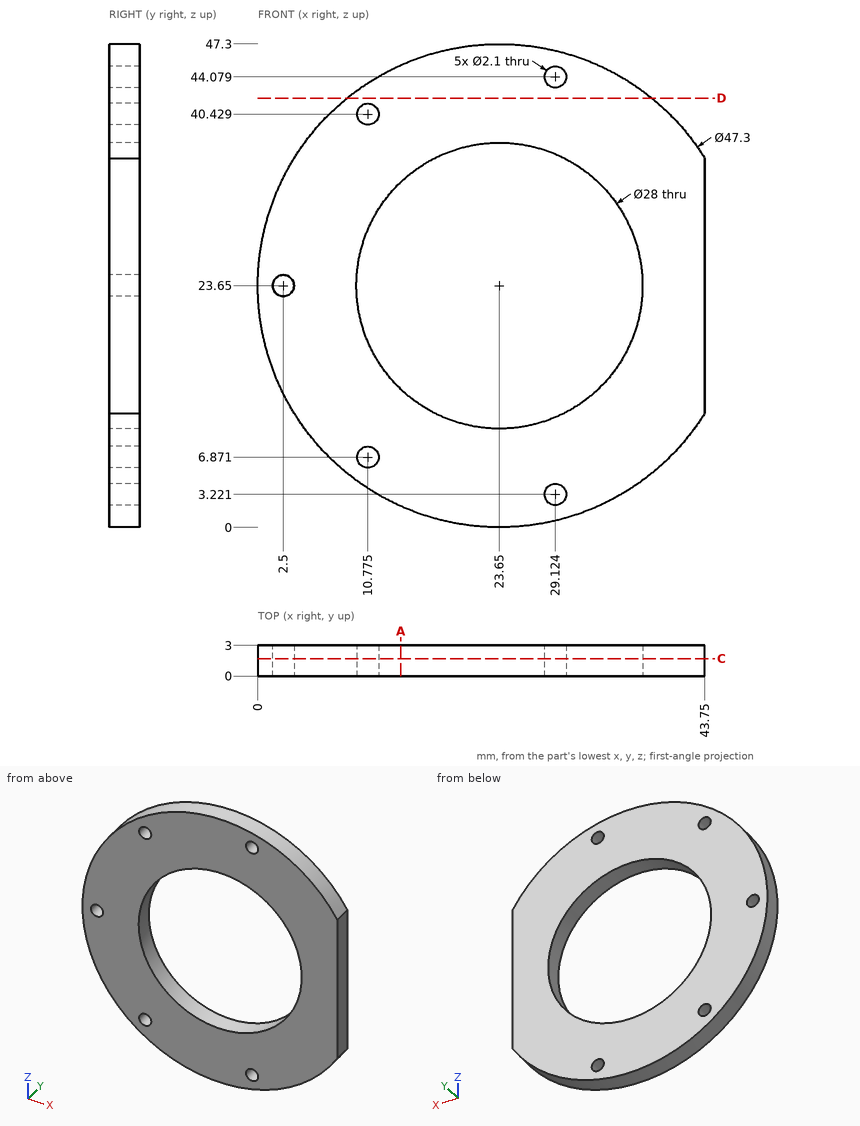
Design review of the part shown in the three views and the two pictorial views. Dimensions are in mm from the part's minimum x, y and z. Coordinates: 2 decimals unless noted, no trailing zeros. Write each loop counter-clockwise with the first axis right and the second up, starting at its lowest first coordinate (ties: lowest second). Pieces come first, ordered by that corner, then holes.
(1) Add section D-D on z = 42. Give the boundary of the cut face in (x, y).
(2) Wall thickness on probe 1 along Z at (x, y) = (20, 0.9) (1 decimal); probe 2 along X at (y, z) = (1.8, 30); probe 3 along X at (y, z) = (1.2, 33.5): over which ranges is each line inside the solid? List them lowest first.
(3) Add section A-A on x = 14. Give the boundary of the cut face in (y, z).
(4) Add section C-C on y = 1.7. Count the separate pieces of the cut face and the enclosed holes in it, then the cut area to 3 significant figures.
(5) For pin 1 Ø4 at (x, z) = (13.5, 12.5) entering from -Y, flat-tipped, find the tip position at first contact; note if it passes through.
Answer sheet:
1. outline: (8.73, 0) - (38.57, 0) - (38.57, 3) - (8.73, 3) - close
2. probe 1: z = 0.3 to 10.1, 37.2 to 47
2. probe 2: x = 0.87 to 11.17, 36.13 to 43.75
2. probe 3: x = 2.15 to 13.7, 33.6 to 43.75
3. outline: (0, 2.06) - (3, 2.06) - (3, 13.51) - (0, 13.51) - close; (0, 33.79) - (3, 33.79) - (3, 45.24) - (0, 45.24) - close
4. separate pieces: 1
4. enclosed holes: 6
4. area: 1,060 mm2
5. pin 1: stops at y = 0
